from build123d import *

# Parameters (mm, degrees)
SKETCH_2_R      = 100
EXTRUDE_1_DEPTH = 15
SKETCH_4_R      = 12.5


with BuildPart() as part:
    # 草图2 → 凸台-拉伸1 (new body)
    with BuildSketch(Plane(origin=(0, 0, 0), x_dir=(1, 0, 0), z_dir=(0, 1, 0))):
        with Locations(Location((0, 0, 0), (0, 0, 270))):
            Circle(SKETCH_2_R)
    extrude(amount=EXTRUDE_1_DEPTH)

    # 扫描1: sweep along a path in 草图3
    with BuildLine(Plane(origin=(0, 0, 0), x_dir=(0, 0, -1), z_dir=(1, 0, 0))) as sweep_1_path:
        Line((73.902769021, 15), (73.902769021, 166.562691704))
        Line((73.902769021, 166.562691704), (73.902769021, 390.709968379))
        ThreePointArc((73.902769021, 390.709968379), (44.192308228, 473.798889435), (-31.466612201, 519.210430284))
    # 草图4 → 扫描1 (sweep)
    with BuildSketch(Plane(origin=(0, 15, 0), x_dir=(1, 0, 0), z_dir=(0, 1, 0))):
        with Locations((0, 73.902769021)):
            Circle(SKETCH_4_R)
    sweep(path=sweep_1_path.line)

    # 草图6 → 旋转1 (revolve)
    with BuildSketch(Plane(origin=(0, 25.969403223, 129.999276708), x_dir=(1, 0, 0), z_dir=(0, 0.19589525539003017, 0.9806248257696085)), mode=Mode.PRIVATE) as revolve_1_sk:
        with BuildLine():
            Line((0, 388.498705936), (0, 591.59882287))
            ThreePointArc((0, 591.59882287), (27.426988969, 583.893568856), (46.828622065, 563.032425634))
            Line((46.828622065, 563.032425634), (46.828622065, 467.578854382))
            add(Edge.make_bspline(
                [(46.828622065, 467.578854382), (47.076936917, 435.310697465), (81.229684313, 420.22666255), (83.059174658, 388.498705936)],
                knots=[0, 0, 0, 0, 1, 1, 1, 1], degree=3))
            Line((83.059174658, 388.498705936), (0, 388.498705936))
        make_face()
    revolve(revolve_1_sk.sketch.rotate(Axis((0, 406.940879043, 53.89422349), (0, 0.9806248257696084, -0.19589525539003022)), 90), axis=Axis((0, 406.940879043, 53.89422349), (0, 0.9806248257696084, -0.19589525539003022)))


solid = part.part
Model file for the job. Use its own axes, mm. Coordinates: 2 decimals unless noted, no trailing zeros. Write each loop counter-clockwise with the first axis right and the second up, starting at its lowest first coordinate (ties: lowest second). Pieces come first, ordered by that corner, then holes. Notation, with made-up numbers: (45.25, -7.75) - (87.25, -7.75) arc R17 ccw to (87.25, 10.25) - close; hole circle Ø3 at (16, -19.75). An arc over 180 degrees is marked (long way). Write each question's results on one line, items separated by ' | '. Start each with the question number.
1) Probe line 1 along Y through (x, z) = (68.5, -68); line 2 along Y through (x, z) = (-42, 30); line 3 along Y through (x, z) = (58, 25). List the from-to ranges inside material, lowest first. Write a range as from..to.
2) Mould opens along Y. For faces 1 (the face through (-1.6, 205.5, -86.3)), 2 (the face through (1, 0, -1)), 3 (the face through (-14.066, 521.886, -14.617)), 4 (the face through (30.04, 7.4, 95.38)) say: pulls with the +Y half, pulls with the -Y half, needs draft (parallel to the pull), parting line crosses it, or undercut.
3) Flat gauge pins, fed straight in: P1, Ø6, axis at x = 27, y = 506, coming from the -Z side; P2, Ø3, axis at x = 9.5, y = 138.5, coming from the -Z side; P3, Ø3, axis at y = 200.5, z = -73, coming from the +X side. Where does each tip first touch, or does it go through?
4) Cut at A-A (y = 270). Write the cut outline in (x, z), then the cut area to 3 significant figures.
Returned:
1) line 1: 0..15 | line 2: 0..15, 402.17..585.74 | line 3: 0..15, 401.17..445.01
2) face 1: undercut | face 2: pulls with the -Y half | face 3: undercut | face 4: needs draft
3) P1: z = -7 | P2: z = -83.51 | P3: x = 12.5
4) outline: circle Ø25 at (0, -73.9) | area: 491 mm^2
